Here's how the part is built. I have some questions about the finished solid (model axes, mm). Face numbers are marked on the shaded views. A direction names the side the tool comes from. Coordinates: 2 decimals unless noted, no trailing zeros. Write each loop counter-clockwise with the first axis right and the second up, starting at its lowest first coordinate (ties: lowest second). Pieces come first, ordered by that corner, then holes.
(1) Imagine slicing it at B-B, the plane x = 0. List the corners of the cut face in (y, z) for me.
(2) Imagine slicing it at C-C, the plane z = -12. List the corners of the cut face in (x, y) for me, plus the area to 3 significant figures.
(3) Which directions (+Z, -Z, +X, -X, +Y, -Y) give clear straight access to the entire face, cutting with the end or side of a thin tool? Please do the marked faces 1 and 2.
(4) Please list where these lines run through material, in increasing order: probe 1 along X at (y, z) = (3.85, 0); probe 2 along Y at (x, z) = (18, 7.5); probe 3 along X at (y, z) = (14.5, 0).
(5) Imagine slicing it at A-A, the plane z = 0. List the corners of the cut face in (x, y) for me.
(6) For pin 1 Ø8 at (y, z) = (9.5, -8) entering from -X; pin 2 Ø2 at (y, z) = (18, -2.5) entering from -X; pin 3 Ø6.5 at (x, z) = (0, 0.5) entering from -Y; pin 4 Ø5 at (x, z) = (0, 0) entering from +Y, each with a flat end and sliding along its axis, tell me the tip position at first contact or that it passes through.
(7) Thinking about a two-plate mould opening in Z: for the marked faces 3, 4 and 5, which applies, released by +Z, released by -Z, zero draft, split by the parting line, or undercut?
(8) Imagine slicing it at D-D, the plane y = 14.5. List the corners of the cut face in (x, z) for me, plus the area to 3 significant figures.
```python
from build123d import *

# Parameters (mm, degrees)
SKETCH_1_R          = 13
EXTRUDE_1_DEPTH     = 20
SKETCH_2_R          = 5.5
CUT_EXTRUDE_2_DEPTH = 5
SKETCH_3_R          = 5
CUT_EXTRUDE_3_DEPTH = 10
CUT_EXTRUDE_3_DRAFT = -7
SKETCH_5_R          = 20
EXTRUDE_7_DEPTH     = 7
SKETCH_7_R          = 3
CUT_EXTRUDE_8_DEPTH = 35.641016151


with BuildPart() as part:
    # Эскиз1 → Вытянуть1 (new body)
    with BuildSketch(Plane(origin=(0, 0, 0), x_dir=(1, 0, 0), z_dir=(0, 1, 0))):
        with Locations(Location((0, 0, 0), (0, 0, 270))):
            Circle(SKETCH_1_R)
    extrude(amount=EXTRUDE_1_DEPTH)

    # Эскиз2 → Вытянуть2 (cut)
    with BuildSketch(Plane.XZ):
        with Locations(Location((0, 0, 0), (0, 0, 270))):
            Circle(SKETCH_2_R)
    extrude(amount=-CUT_EXTRUDE_2_DEPTH, mode=Mode.SUBTRACT)


with BuildPart() as cut_extrude_3_tool:
    # Эскиз3 → Вытянуть3 (with draft: the straight prism first)
    with BuildSketch(Plane.XZ.offset(-5)):
        Circle(SKETCH_3_R)
    extrude(amount=-CUT_EXTRUDE_3_DEPTH)
    # Вытянуть3: the draft: its side faces are tilted about the plane it starts from
    cut_extrude_3_sides = [cut_extrude_3_tool.faces().sort_by_distance(p)[0] for p in [
        (-5, 10, 0),
    ]]
    draft(cut_extrude_3_sides, Plane.XZ.offset(-5), CUT_EXTRUDE_3_DRAFT)


with BuildPart() as part_1:
    add(part.part)

    # Вытянуть3: cut by cut_extrude_3_tool
    add(cut_extrude_3_tool.part, mode=Mode.SUBTRACT)

    # Эскиз5 → Вытянуть7 (add)
    with BuildSketch(Plane(origin=(0, 20, 0), x_dir=(-1, 0, 0), z_dir=(0, 1, 0))):
        with Locations(Location((0, 0, 0), (0, 0, 90))):
            Circle(SKETCH_5_R)
    extrude(amount=-EXTRUDE_7_DEPTH)

    # Эскиз7 → Вытянуть8 (cut, through all)
    with BuildSketch(Plane(origin=(0, 20, 0), x_dir=(1, 0, 0), z_dir=(0, 1, 0))):
        with Locations(Location((0, 0, 0), (0, 0, 270))):
            Circle(SKETCH_7_R)
    extrude(amount=-CUT_EXTRUDE_8_DEPTH, mode=Mode.SUBTRACT)


solid = part_1.part
```
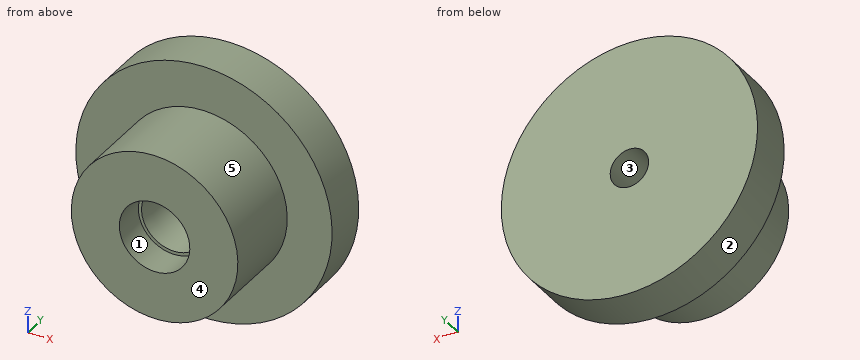
Recorded:
1. outline: (0, -13) - (13, -13) - (13, -20) - (20, -20) - (20, -3) - (13, -3) - (13, -4.02) - (5, -5) - (5, -5.5) - (0, -5.5) - close; (0, 5.5) - (5, 5.5) - (5, 5) - (13, 4.02) - (13, 3) - (20, 3) - (20, 20) - (13, 20) - (13, 13) - (0, 13) - close
2. outline: (-16, 13) - (-5, 13) - (-5, 0) - (5, 0) - (5, 13) - (16, 13) - (16, 20) - (-16, 20) - close
2. area: 354 mm2
3. face 1: -Y
3. face 2: +Y, -Y
4. probe 1: x = -13 to -5.5, 5.5 to 13
4. probe 2: y = 13 to 20
4. probe 3: x = -20 to -3, 3 to 20
5. outline: (-20, 13) - (-13, 13) - (-13, 0) - (-5.5, 0) - (-5.5, 5) - (-5, 5) - (-4.02, 13) - (-3, 13) - (-3, 20) - (-20, 20) - close; (3, 13) - (4.02, 13) - (5, 5) - (5.5, 5) - (5.5, 0) - (13, 0) - (13, 13) - (20, 13) - (20, 20) - (3, 20) - close
6. pin 1: stops at x = -19.06
6. pin 2: stops at x = -19.94
6. pin 3: stops at y = 13
6. pin 4: passes through
7. face 3: undercut
7. face 4: zero draft
7. face 5: split by the parting line
8. outline: circle Ø40 at (0, 0); hole circle Ø6 at (0, 0)
8. area: 1,230 mm2
